For this review, use the dimensioned drawing (mm, ordinates from the lowest corner) and the shaded views. A direction names the side the tool comes from. Coordinates: 2 decimals unless noted, no trailing zeros. Loops run counter-clockwise (first coordinate to the right, second up) from the corner with the lowest first, then second, coordinate; pieces in that order, holes last. Notation, with made-up numbers: M 64,86 L 84,86 A20 ccw 84,108 Z; hole C 1.5,6.25 d7. An arc over 180 degrees is marked long. One line per item, written item: value.
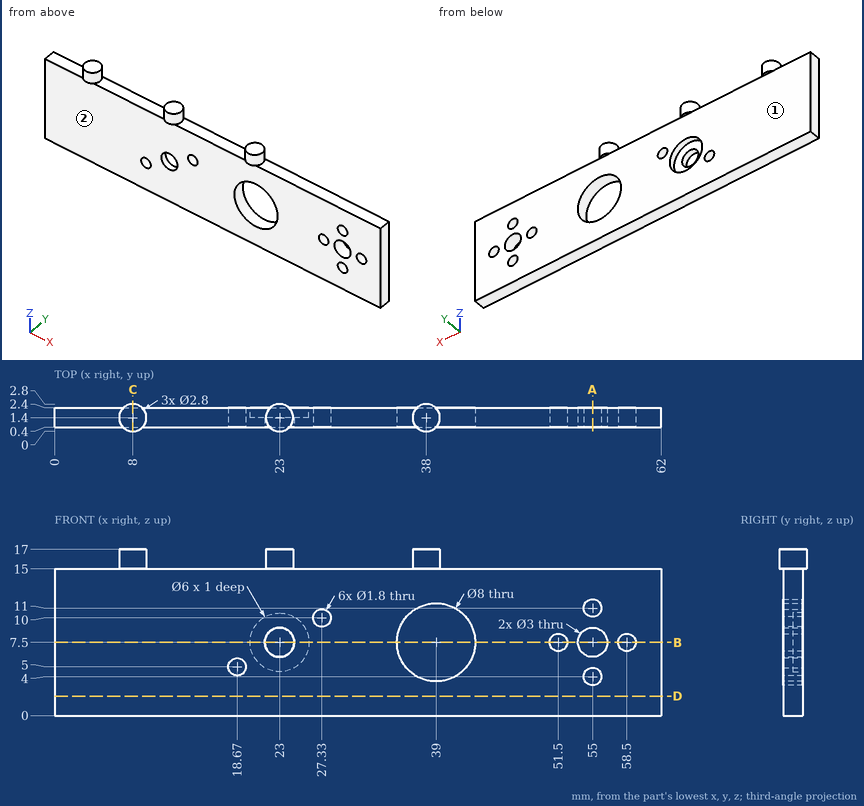
(1) Tool access review of the marked faces 1 and 2: name each direction out of +Z, -Z, +X, -X, +Y, -Y from which nothing blocks a thin tool from reaching the whole face with its end or side.
Reply:
face 1: -Z, +X, -X, +Y
face 2: -Z, +X, -X, -Y
(2) We need section C-C on x = 8. State the section outline as (y, z) points.
Reply:
outline: M 0,15 L 0.4,15 L 0.4,0 L 2.4,0 L 2.4,15 L 2.8,15 L 2.8,17 L 0,17 Z
(3) We need section D-D on z = 2. State the section outline as (x, y) points, then the cut area to 3 significant figures.
Reply:
outline: M 0,0.4 L 62,0.4 L 62,2.4 L 0,2.4 Z
area: 124 mm2
(4) We need section B-B on z = 7.5. State the section outline as (x, y) points, then the cut area to 3 significant figures.
Reply:
outline: M 0,0.4 L 21.5,0.4 L 21.5,1.4 L 20,1.4 L 20,2.4 L 0,2.4 Z; M 24.5,0.4 L 35,0.4 L 35,2.4 L 26,2.4 L 26,1.4 L 24.5,1.4 Z; M 43,0.4 L 50.6,0.4 L 50.6,2.4 L 43,2.4 Z; M 52.4,0.4 L 53.5,0.4 L 53.5,2.4 L 52.4,2.4 Z; M 56.5,0.4 L 57.6,0.4 L 57.6,2.4 L 56.5,2.4 Z; M 59.4,0.4 L 62,0.4 L 62,2.4 L 59.4,2.4 Z
area: 85.8 mm2
(5) Insertion check: pin 1 (6 mm diameter, centred on x = 55, z = 13, fed in from -Y); pin 2 (7.5 mm diameter, centred on x = 24, z = 7.5, fed in from +Y); pin 3 (1.6 mm diameter, centred on x = 12.5, y = 1.5, fed in from +Z); pin 4 (1.1 mm diameter, centred on x = 58.5, z = 7.5, fed in from +Y). Each pin has a flat end and moves straight along its axis. Give the tip position at first contact, or say it passes through.
Reply:
pin 1: stops at y = 0.4
pin 2: stops at y = 2.4
pin 3: stops at z = 15
pin 4: passes through
(6) To check wall thickness, follow line 1 along Z through (x, y) = (51.5, 1.6); line 2 along X through (y, z) = (1.5, 7.5); line 3 along Z through (x, y) = (16, 1.15). State the ranges of each line that lie inside material, in increasing order. Write a range as [from, to].
Reply:
line 1: z = [0, 6.6], [8.4, 15]
line 2: x = [0, 20], [26, 35], [43, 50.6], [52.4, 53.5], [56.5, 57.6], [59.4, 62]
line 3: z = [0, 15]
(7) We need section A-A on x = 55. State the section outline as (y, z) points.
Reply:
outline: M 0.4,0 L 2.4,0 L 2.4,3.1 L 0.4,3.1 Z; M 0.4,4.9 L 2.4,4.9 L 2.4,6 L 0.4,6 Z; M 0.4,9 L 2.4,9 L 2.4,10.1 L 0.4,10.1 Z; M 0.4,11.9 L 2.4,11.9 L 2.4,15 L 0.4,15 Z
